Build history of the part. All positions in model axes, mm. Give positions to 0.01 mm unless a question says otherwise; leave off trailing zeros. Loops run counter-clockwise (first coordinate to the right, second up) from the corner with the lowest first, then second, coordinate; pieces in that order, holes last.
1) Band-saw the part on B-B on z = 15. List the corners of the cut face in (x, y).
2) Band-saw the part on A-A on x = -18. State how many separate pieces and enclosed holes the cut face has, then the cut area to 3 significant figures.
3) Flat gauge pins, fed straight in: P1, Ø12, axis at x = -26.5, y = 15, coming from the +Z side; P2, Ø23, axis at x = -59, y = 33, coming from the +Z side; P3, Ø20.5, axis at x = -18, y = -680, coming from the -Z side; P4, Ø4, axis at x = -38.5, y = -504.5, coming from the -Z side. Where does each tip first touch, or does it go through?
4) Wall check: line 1 (Y direction, x = -18, z = 1.35); line 2 (X direction, y = -720, z = 1); line 3 (Z direction, x = -19, y = -230). Give the ranges that are in metal, low to high.
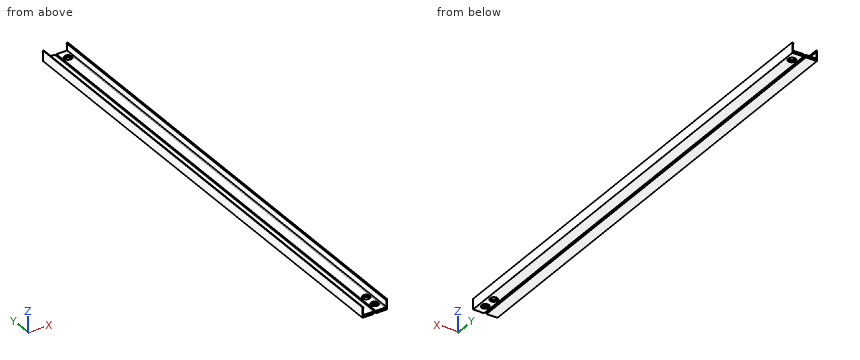
```python
from build123d import *

# Parameters (mm, degrees)
F1_DEPTH = 750
F2_R     = 0.5
F3_R     = 11.5
F4_DEPTH = 25.4


with BuildPart() as f1:
    # F0 (on Front) → F1 (new body, symmetric)
    with BuildSketch(Plane.XZ):
        Polygon((-0.121622, 0), (0, 0), (0, 32), (-2, 32), (-2, 30), (-3.631513, 30), (-3.744032, 28.255974), (-2, 26.399431), (-2.397815, 9.028868), (-5.717093, 7.453618), (-34.352882, 7.453618), (-36.09691, 5.372039), (-39.544148, 5.372039), (-41.288176, 7.453618), (-69.923965, 7.453618), (-73.243243, 9.028868), (-73.243243, 26.525391), (-71.499211, 28.381934), (-71.61173, 30), (-73.243243, 30), (-73.243243, 32), (-75.243243, 32), (-75.243243, 0), (-41.003749, 0), (-41.003749, 1.284304), (-43.03767, 1.311418), (-43.149501, 5.337393), (-42.076625, 5.367195), (-41.063354, 4.085704), (-37.743243, 4.085704), (-34.301511, 4.085704), (-33.28824, 5.367195), (-32.215363, 5.337393), (-32.327195, 1.311418), (-34.361116, 1.284304), (-34.361116, 0), align=None)
        Polygon((-44.694386, 5.337393), (-44.694386, 1.910149), (-73.364027, 1.910149), (-73.393829, 2.506191), (-71.754345, 2.588166), (-71.789201, 3.285283), (-73.542841, 3.638672), (-73.202291, 5.328597), (-71.605705, 5.665216), (-70.68184, 4.502933), (-69.936782, 5.337393), align=None, mode=Mode.SUBTRACT)
        Polygon((-3.637539, 5.665216), (-2.040952, 5.328597), (-1.700402, 3.638672), (-3.454042, 3.285283), (-3.488898, 2.588166), (-1.849414, 2.506191), (-1.879216, 1.910149), (-30.548857, 1.910149), (-30.548857, 5.337393), (-5.306461, 5.337393), (-4.561403, 4.502933), align=None, mode=Mode.SUBTRACT)
    extrude(amount=F1_DEPTH, both=True)

    # F2
    f2_edges = [f1.edges().sort_by_distance(p)[0] for p in [
        (-75.243243, 0, 32),
        (0, 0, 32),
        (0, 0, 0),
        (-75.243243, 0, 0),
        (-41.003749, 0, 0),
        (-34.361116, 0, 0),
    ]]
    fillet(f2_edges, radius=F2_R)

    # F3 (on face) → F4 (cut)
    with BuildSketch(Plane.XY.offset(7.453618)):
        with Locations((-18, -720)):
            Circle(F3_R)
        with Locations((-18, -680)):
            Circle(F3_R)
        with Locations((-18, 720)):
            Circle(F3_R)
    extrude(amount=-F4_DEPTH, mode=Mode.SUBTRACT)


solid = f1.part
```
Findings below:
1. outline: (-75.24, -750) - (-73.24, -750) - (-73.24, 750) - (-75.24, 750) - close; (-2.26, -750) - (0, -750) - (0, 750) - (-2.26, 750) - close
2. separate pieces: 8
2. enclosed holes: 0
2. area: 5,760 mm2
3. P1: stops at z = 7.45
3. P2: stops at z = 7.73
3. P3: passes through
3. P4: stops at z = 4.09
4. line 1: y = -750 to -731.5, -708.5 to -691.5, -668.5 to 708.5, 731.5 to 750
4. line 2: x = -75.24 to -41, -34.36 to -29.5, -6.5 to 0
4. line 3: z = 0 to 1.91, 5.34 to 7.45
